Design review of the part built by this model. Coordinates are the model's own, in mm. A direction names the side the tool comes from. Coordinates: 2 decimals unless noted, no trailing zeros. Order: outer loops, then holes, each group sorted by start corner. A loop starts at its lowest first (then second) coordinate and runs counter-clockwise, first axis right, second up. Notation, with made-up numbers: M -32.75,51.25 L 2.25,51.25 A12 cw 2.25,70.25 Z; hole C 61,-24.75 d5. An arc over 180 degrees is marked long. Use CSV: the item, a comma, the result in double quotes.
Autodesk Fusion 360 part; units mm, degrees
sketch "Sketch1" plane through (0, 0, 0) normal (0, 0, 1) x (1, 0, 0)
  line L0 (0, 0) -> (17.9, 0)
  line L1 (17.9, 0) -> (17.9, 10.8)
  line L2 (17.9, 10.8) -> (0, 10.8)
  line L3 (0, 10.8) -> (0, 0)
  dimension "d1" = 17.9
  dimension "d2" = 10.8
extrude "Extrude1" add sketch "Sketch1" along normal blind 7.9
chamfer "Chamfer1" distance 2.2 angle 45 2 edges at (8.95, 10.8, 7.9) (8.95, 0, 7.9)
sketch "Sketch2" plane through (0, 0, 0) normal (-1, 0, 0) x (0, -1, 0)
  line L0 (0, 5.7) -> (-2.2, 7.9)
  line L1 (-2.2, 7.9) -> (-8.6, 7.9)
  line L2 (-8.6, 7.9) -> (-10.8, 5.7)
  line L3 (-10.8, 5.7) -> (-10.8, 0)
  line L4 (-10.8, 0) -> (0, 0)
  line L5 (0, 0) -> (0, 5.7)
  line L6 (-5.4, 7.9) -> (-5.4, 0) construction
  line L7 (-5.4, 3.95) -> (0, 3.95) construction
  line L8 (-2, 3.05) -> (-8.8, 3.05)
  line L9 (-8.8, 3.05) -> (-8.8, 4.85)
  line L10 (-8.8, 4.85) -> (-2, 4.85)
  line L11 (-2, 4.85) -> (-2, 3.05)
  line L12 (-2, 3.05) -> (-8.8, 4.85) construction
  line L13 (-8.8, 3.05) -> (-2, 4.85) construction
  point P0 (-5.4, 3.95)
  dimension "d6" = 6.8
  dimension "d7" = 1.8
extrude "Extrude2" add sketch "Sketch2" along normal blind 6 contours L8 L9 L10 L11
chamfer "Chamfer2" distance 1 angle 45 2 edges at (-3, 8.8, 3.05) (-3, 2, 3.05)
sketch "Sketch3" plane through (17.9, 0, 0) normal (1, 0, 0) x (0, 1, 0)
  line L0 (2.2, 7.9) -> (0, 5.7)
  line L1 (0, 5.7) -> (0, 0)
  line L2 (0, 0) -> (10.8, 0)
  line L3 (10.8, 0) -> (10.8, 5.7)
  line L4 (10.8, 5.7) -> (8.6, 7.9)
  line L5 (8.6, 7.9) -> (2.2, 7.9)
  line L6 (5.4, 7.9) -> (5.4, 0) construction
  line L7 (5.4, 3.95) -> (10.8, 3.95) construction
  line L8 (9.2, 0.85) -> (1.6, 0.85)
  line L9 (1.6, 0.85) -> (1.6, 7.05)
  line L10 (1.6, 7.05) -> (9.2, 7.05)
  line L11 (9.2, 7.05) -> (9.2, 0.85)
  line L12 (9.2, 0.85) -> (1.6, 7.05) construction
  line L13 (1.6, 0.85) -> (9.2, 7.05) construction
  point P0 (5.4, 3.95)
  dimension "d11" = 6.2
  dimension "d12" = 7.6
extrude "Extrude3" add sketch "Sketch3" along normal blind 12 draft -3 contours L8 L9 L10 L11
sketch "Sketch4" plane through (29.9, 0, 0) normal (1, 0, 0) x (0, 1, 0)
  line L0 (8.5711, 1.4789) -> (8.5711, 6.4211)
  line L1 (8.5711, 6.4211) -> (2.2289, 6.4211)
  line L2 (2.2289, 6.4211) -> (2.2289, 1.4789)
  line L3 (2.2289, 1.4789) -> (8.5711, 1.4789)
  line L4 (5.4, 6.4211) -> (5.4, 1.4789) construction
  line L5 (2.2289, 3.95) -> (8.5711, 3.95) construction
  circle A0 centre (5.4, 3.95) radius 1.9
  dimension "d15" = 3.8
extrude "Extrude4" add sketch "Sketch4" along normal blind 18 contours A0
fillet "Fillet1" radius 1 4 edges at (23.9, 1.9144, 6.7356) (23.9, 8.8856, 6.7356) (23.9, 1.9144, 1.1644) (23.9, 8.8856, 1.1644)
(1) Add section B-B on y = 5.4. State the section outline as (x, z) points, and give its area (3 significant figures).
The answers:
outline,"M -6,3.05 L 0,3.05 L 0,0 L 17.9,0 L 17.9,0.85 L 29.9,1.48 L 29.9,2.05 L 47.9,2.05 L 47.9,5.85 L 29.9,5.85 L 29.9,6.42 L 17.9,7.05 L 17.9,7.9 L 0,7.9 L 0,4.85 L -6,4.85 Z"
area,"287 mm2"
(2) The part is to be moulded in two halves that separate along X. For faces 1 (the face through (9.1, 1.1, 6.8)), 2 (the face through (-6, 5, 4)), 3 (the face through (29.9, 7.5, 4)), say which applies: pulls with the +X half, pulls with the -X half, needs draft (parallel to the pull), parting line crosses it, or undercut.
The answers:
face 1,"needs draft"
face 2,"pulls with the -X half"
face 3,"pulls with the +X half"
(3) Clearance check with flat-ended pins moving along their axes: P1, Ø5, axis at x = 38.5, y = 6, coming from the +Z side; P2, Ø2.5, axis at x = -4.5, y = 4.5, coming from the -Z side; P3, Ø4, axis at x = 28.5, z = 4.5, coming from the -Y side. State where each tip first meets the part, or that it passes through.
The answers:
P1,"stops at z = 5.85"
P2,"stops at z = 3.05"
P3,"stops at y = 2.05"
(4) For faces 4 (the face through (-3, 5, 4.85)), 5 (the face through (-2.96, 8.31, 3.56)), 6 (the face through (-3.04, 2.49, 3.56)), 7 (the face through (17.9, 5, 0.7)), 8 (the face through (23.82, 5.44, 1.16)), list the 3-axis set-ups (+Z, -Z, +X, -X, +Y, -Y) from which the entire face can be reached by the end or side of a thin tool; tool diameter is ignored.
The answers:
face 4,"+Z, -X, +Y, -Y"
face 5,"-Z, -X, +Y"
face 6,"-Z, -X, -Y"
face 7,"+X"
face 8,"-Z, +X, +Y, -Y"
(5) Add section A-A on x = 17. State the section outline as (y, z) points.
The answers:
outline,"M 0,0 L 10.8,0 L 10.8,5.7 L 8.6,7.9 L 2.2,7.9 L 0,5.7 Z"
(6) Add section C-C on x = 39.5. State the section outline as (y, z) points.
The answers:
outline,"C 5.4,3.95 d3.8"
(7) Wall thickness on probe 1 along X at (y, z) = (8, 2.5); probe 2 along X at (y, z) = (1, 5.5); probe 3 along Y at (x, z) = (34, 4): over which ranges is each line inside the solid? List them lowest first.
The answers:
probe 1,"x = 0 to 29.9"
probe 2,"x = 0 to 17.9"
probe 3,"y = 3.5 to 7.3"
